from build123d import *

# Parameters (mm, degrees)
F1_DEPTH = 6.9342


with BuildPart() as f1:
    # F0 (on Front) → F1 (new body)
    with BuildSketch(Plane.XZ):
        with BuildLine():
            Line((28.202122, 22.984592), (9.230435, 12.031283))
            ThreePointArc((9.230435, 12.031283), (8.177557, 12.772114), (7.065545, 13.420814))
            Line((7.065545, 13.420814), (7.065545, 33.731301))
            ThreePointArc((7.065545, 33.731301), (0.758717, 52.689846), (-5.54811, 33.731301))
            Line((-5.54811, 33.731301), (-5.54811, 14.117454))
            ThreePointArc((-5.54811, 14.117454), (-6.591857, 13.660258), (-7.59826, 13.125854))
            Line((-7.59826, 13.125854), (-26.438109, 24.003046))
            ThreePointArc((-26.438109, 24.003046), (-46.010104, 28.020445), (-32.744936, 13.0793))
            Line((-32.744936, 13.0793), (-15.183252, 2.940057))
            Line((-15.183252, 2.940057), (-14.407735, -1.035813))
            Line((-14.407735, -1.035813), (-33.247584, -11.913005))
            ThreePointArc((-33.247584, -11.913005), (-46.512752, -26.85415), (-26.940757, -22.83675))
            Line((-26.940757, -22.83675), (-9.379072, -12.697507))
            Line((-9.379072, -12.697507), (-6.306827, -13.731525))
            Line((-6.306827, -13.731525), (-6.306827, -34.749755))
            ThreePointArc((-6.306827, -34.749755), (0, -53.7083), (6.306827, -34.749755))
            Line((6.306827, -34.749755), (6.306827, -13.731525))
            Line((6.306827, -13.731525), (7.59826, -13.125854))
            Line((7.59826, -13.125854), (26.438109, -24.003046))
            ThreePointArc((26.438109, -24.003046), (46.010104, -28.020445), (32.744936, -13.0793))
            Line((32.744936, -13.0793), (15.183252, -2.940057))
            Line((15.183252, -2.940057), (16.33474, 1.567961))
            Line((16.33474, 1.567961), (34.50895, 12.060847))
            ThreePointArc((34.50895, 12.060847), (47.774118, 27.001992), (28.202122, 22.984592))
        make_face()
        with BuildLine():
            ThreePointArc((6.306827, -42.440791), (6.339198, -42.809766), (6.35, -43.18))
            ThreePointArc((6.35, -43.18), (6.339198, -43.550234), (6.306827, -43.919209))
            ThreePointArc((6.306827, -43.919209), (0, -49.53), (-6.306827, -43.919209))
            ThreePointArc((-6.306827, -43.919209), (-6.35, -43.18), (-6.306827, -42.440791))
            ThreePointArc((-6.306827, -42.440791), (0, -36.83), (6.306827, -42.440791))
        make_face(mode=Mode.SUBTRACT)
        with BuildLine():
            ThreePointArc((-34.881737, -27.421477), (-42.894238, -24.765), (-41.188564, -16.497732))
            ThreePointArc((-41.188564, -16.497732), (-40.569977, -16.090739), (-39.908217, -15.758523))
            ThreePointArc((-39.908217, -15.758523), (-33.904746, -16.285211), (-31.044977, -21.59))
            ThreePointArc((-31.044977, -21.59), (-31.719954, -24.438967), (-33.60139, -26.682268))
            ThreePointArc((-33.60139, -26.682268), (-34.219977, -27.089261), (-34.881737, -27.421477))
        make_face(mode=Mode.SUBTRACT)
        with BuildLine():
            ThreePointArc((43.242329, -22.756295), (40.38256, -28.061085), (34.379089, -28.587772))
            ThreePointArc((34.379089, -28.587772), (33.717329, -28.255557), (33.098742, -27.848564))
            ThreePointArc((33.098742, -27.848564), (31.393068, -19.581295), (39.405569, -16.924818))
            ThreePointArc((39.405569, -16.924818), (40.067329, -17.257034), (40.685916, -17.664027))
            ThreePointArc((40.685916, -17.664027), (42.567352, -19.907329), (43.242329, -22.756295))
        make_face(mode=Mode.SUBTRACT)
        with BuildLine():
            ThreePointArc((-33.098742, 27.848564), (-31.217306, 25.605262), (-30.542329, 22.756295))
            ThreePointArc((-30.542329, 22.756295), (-33.402098, 17.451506), (-39.405569, 16.924818))
            ThreePointArc((-39.405569, 16.924818), (-40.067329, 17.257034), (-40.685916, 17.664027))
            ThreePointArc((-40.685916, 17.664027), (-42.39159, 25.931295), (-34.379089, 28.587772))
            ThreePointArc((-34.379089, 28.587772), (-33.717329, 28.255557), (-33.098742, 27.848564))
        make_face(mode=Mode.SUBTRACT)
        with BuildLine():
            ThreePointArc((5.319741, 9.773443), (9.546036, 5.695287), (11.0998, 0.031477))
            ThreePointArc((11.0998, 0.031477), (11.072628, -0.744715), (10.991244, -1.517107))
            ThreePointArc((10.991244, -1.517107), (-1.047034, -11.01883), (-11.086495, 0.574793))
            ThreePointArc((-11.086495, 0.574793), (-8.770532, 6.834662), (-3.28325, 10.634581))
            ThreePointArc((-3.28325, 10.634581), (1.105538, 11.076084), (5.319741, 9.773443))
        make_face(mode=Mode.SUBTRACT)
        with BuildLine():
            ThreePointArc((36.143102, 27.569319), (42.146573, 27.042631), (45.006342, 21.737842))
            ThreePointArc((45.006342, 21.737842), (44.331366, 18.888875), (42.449929, 16.645573))
            ThreePointArc((42.449929, 16.645573), (41.831342, 16.23858), (41.169583, 15.906365))
            ThreePointArc((41.169583, 15.906365), (33.157081, 18.562842), (34.862755, 26.83011))
            ThreePointArc((34.862755, 26.83011), (35.481342, 27.237103), (36.143102, 27.569319))
        make_face(mode=Mode.SUBTRACT)
        with BuildLine():
            ThreePointArc((-5.54811, 42.900755), (0.758717, 48.511546), (7.065545, 42.900755))
            ThreePointArc((7.065545, 42.900755), (7.097915, 42.53178), (7.108717, 42.161546))
            ThreePointArc((7.108717, 42.161546), (7.097915, 41.791312), (7.065545, 41.422338))
            ThreePointArc((7.065545, 41.422338), (0.758717, 35.811546), (-5.54811, 41.422338))
            ThreePointArc((-5.54811, 41.422338), (-5.591283, 42.161546), (-5.54811, 42.900755))
        make_face(mode=Mode.SUBTRACT)
    extrude(amount=F1_DEPTH)


solid = f1.part
Work out the finished part from the listing and answer in its coordinate system (mm). Give positions to 0.01 mm unless a question says otherwise; leave off trailing zeros. Loops run counter-clockwise (first coordinate to the right, second up) from the corner with the lowest first, then second, coordinate; pieces in that order, holes last. Notation, with made-up numbers: M 61.25,-25 L 118.25,-25 A18 ccw 118.25,2 Z; hole C -36.5,-25 d1. An arc over 180 degrees is marked long. Use CSV: the item, a comma, the result in double quotes.
1) Find section A-A on x = 3. Write down the section's boundary in (y, z), plus the area to 3 significant figures.
Answer:
outline,"M -6.93,-53.27 L 0,-53.27 L 0,-48.78 L -6.93,-48.78 Z; M -6.93,-37.58 L 0,-37.58 L 0,-10.66 L -6.93,-10.66 Z; M -6.93,10.72 L 0,10.72 L 0,36.22 L -6.93,36.22 Z; M -6.93,48.1 L 0,48.1 L 0,52.45 L -6.93,52.45 Z"
area,"425 mm^2"
2) Consider L1, parallel to Z at x = 3, y = -5.5; L2, parallel to X at y = -3.25, z = 17.5; L3, parallel to X at y = -1.25, z = 13.5. Determine where each line is inside the solid, lowest interval first.
Answer:
L1,"-53.27 to -48.78, -37.58 to -10.66, 10.72 to 36.22, 48.1 to 52.45"
L2,"-46.01 to -40.46, -33.33 to -15.17, -5.55 to 7.07, 18.7 to 33.93, 43.39 to 48.29"
L3,"-41.91 to -8.25, -6.91 to 7.07, 11.77 to 45.21"
3) Determine the mould class of faces 1 (the cylindrical face through (-42.455, -3.419, 25.819)), 2 (the flat face through (-3, -6.934, 12)), 3 (the cylindrical face through (-0.4, -3.4, -53.7)) for opening direction X: released by +X, released by -X, zero draft, split by the parting line, or undercut.
Answer:
face 1,"undercut"
face 2,"zero draft"
face 3,"split by the parting line"
4) Find section C-C on x = -23. Write down the section's boundary in (y, z).
Answer:
outline,"M -6.93,-20.56 L 0,-20.56 L 0,-6 L -6.93,-6 Z; M -6.93,7.45 L 0,7.45 L 0,22.02 L -6.93,22.02 Z"
5) Find section D-D on y = -5. Give the number of separate pieces and of enclosed holes in the cut face, plus the area to 3 significant figures.
Answer:
separate pieces,"1"
enclosed holes,"7"
area,"3,080 mm^2"
6) Find section B-B on z = -8.5. Write down the section's boundary in (x, y).
Answer:
outline,"M -27.34,-6.93 L -7.1,-6.93 L -7.1,0 L -27.34,0 Z; M 7.1,-6.93 L 24.81,-6.93 L 24.81,0 L 7.1,0 Z"
7) Given P1, Ø3.5, axis at y = -5, z = 22.5, coming from the -X side; P2, Ø1.5, axis at x = -37.5, y = -5, coming from the -Z side; P3, Ø3, axis at y = -4, z = -15.5, coming from the +X side, each flat-ended and moving along its own axis, determine where each tip first touches the part or whether it passes through.
Answer:
P1,"x = -47.42"
P2,"z = -32.12"
P3,"x = 45.71"
